The listing builds one solid part. Answer for the finished solid, in the listing's coordinates (mm). A direction names the side the tool comes from. Round coordinates to 2 decimals unless told otherwise and drop trailing zeros. Write each loop counter-clockwise with the first axis right and the second up, starting at its lowest first coordinate (ties: lowest second). Pieces come first, ordered by that corner, then holes. Notation, with made-up numbers: (-38, 76) - (1, 76) arc R24 ccw to (1, 90) - close; hole circle Ø11 at (80.25, 69.25). An arc over 180 degrees is marked (long way). Return JSON: item names as keys, results as strings. Group by question number.
(1) Determine the mould class of faces 1 (the cylindrical face through (54.46, 6.09, -1.48)), 2 (the flat face through (0, 0, -47)), 3 (the flat face through (59, 6, -3)) for opening direction Y: +Y half, -Y half, draft (parallel to the pull), parting line (faces both ways), or undercut.
(2) Section A-A, the plane y = 6 is taken. Write down the section's boundary in (x, z), then the cut area to 3 significant figures.
(3) Which of the six approach directions +Z, -Z, +X, -X, +Y, -Y give full straight-line access (tool end or side, diameter ignored) to faces 4 (the flat face through (-59, 6, -3)), 5 (the flat face through (-61.5, 6, -2))?
(4) Section C-C, the plane x = 0 is taken. Write down the section's boundary in (y, z), then the cut area to 3 significant figures.
(5) Find the intervals of material crossed by line 1 along Z through (x, y) = (57, 8); line 2 along X through (y, z) = (9, -1.5); line 3 along X through (y, z) = (6, -6), in increasing order. Write a range as [from, to].
(6) Section D-D, the plane x = 28 is taken. Write down the section's boundary in (y, z).
(7) Section B-B, the plane z = -24 is taken. Write down the section's boundary in (x, y).
(8) Each of these flat-tipped pins is pushed along its axis until it touches: pin 1 (3 mm diameter, centred on x = 22, y = 2.5, fed in from +Z); pin 2 (1.5 mm diameter, centred on x = 13, y = 8.5, fed in from -Z); pin 3 (2 mm diameter, centred on y = 8.5, z = -27, fed in from +X). Where does it stop, or does it pass through?
```python
from build123d import *

# Parameters (mm, degrees)
SKETCH1_R           = 46.5
BOSS_EXTRUDE1_DEPTH = 12
SKETCH2_R           = 2
CUT_EXTRUDE1_DEPTH  = 12
SKETCH3_W           = 95
SKETCH3_H           = 5
BOSS_EXTRUDE2_DEPTH = 12
MOVE_FACE1_BY       = 3
MOVE_FACE2_BY       = 3
MOVE_FACE2_2_BY     = 3
SKETCH4_R           = 2
CUT_EXTRUDE2_DEPTH  = 114.80355882
CUT_EXTRUDE3_DEPTH  = 2
FILLET1_R           = 1
FILLET2_R           = 1


with BuildPart() as part:
    # Sketch1 → Boss-Extrude1 (new body)
    with BuildSketch(Plane(origin=(0, 0, 0), x_dir=(1, 0, 0), z_dir=(0, 1, 0))):
        with BuildLine():
            Line((61.5, -3), (61.5, 3))
            Line((61.5, 3), (51.412547107, 3))
            ThreePointArc((51.412547107, 3), (0, 51.5), (-51.412547107, 3))
            Line((-51.412547107, 3), (-61.5, 3))
            Line((-61.5, 3), (-61.5, -3))
            Line((-61.5, -3), (-51.412547107, -3))
            ThreePointArc((-51.412547107, -3), (0, -51.5), (51.412547107, -3))
            Line((51.412547107, -3), (61.5, -3))
        make_face()
        with Locations(Location((0, 0, 0), (0, 0, 270))):
            Circle(SKETCH1_R, mode=Mode.SUBTRACT)
    extrude(amount=BOSS_EXTRUDE1_DEPTH)

    # Sketch2 → Cut-Extrude1 (cut)
    with BuildSketch(Plane.XY.offset(3)):
        with Locations((56.456273553, 6)):
            Circle(SKETCH2_R)
        with Locations((-56.456273553, 6)):
            Circle(SKETCH2_R)
    extrude(amount=-CUT_EXTRUDE1_DEPTH, mode=Mode.SUBTRACT)


with BuildPart() as body_2:
    # Split1: the piece on the far side of the plane
    add(part.part)
    split(bisect_by=Plane.XY, keep=Keep.BOTTOM)

    # Fillet2
    fillet2_edges = [body_2.edges().sort_by_distance(p)[0] for p in [
        (51.412547107, 6, -3),
        (-51.412547107, 6, -3),
    ]]
    fillet(fillet2_edges, radius=FILLET2_R)


with BuildPart() as part_1:
    add(part.part)

    # Split1
    split(bisect_by=Plane.XY, keep=Keep.TOP)

    # Sketch3 → Boss-Extrude2 (add)
    with BuildSketch(Plane(origin=(0, 12, 0), x_dir=(1, 0, 0), z_dir=(0, 1, 0))):
        with Locations((0, -49)):
            Rectangle(SKETCH3_W, SKETCH3_H)
    extrude(amount=-BOSS_EXTRUDE2_DEPTH)

    # Move Face1: a face moved inward by 3.0
    extrude(part_1.faces().sort_by_distance((0, 6, 51.5))[0], amount=MOVE_FACE1_BY, dir=(0, 0, -1), mode=Mode.SUBTRACT)

    # Move Face2: a face moved outward by 3.0
    extrude(part_1.faces().sort_by_distance((34.817971811, 6, 46.5))[0], amount=MOVE_FACE2_BY, dir=(0, 0, -1))

    # Move Face2 2: a face moved outward by 3.0
    extrude(part_1.faces().sort_by_distance((-34.817971811, 6, 46.5))[0], amount=MOVE_FACE2_2_BY, dir=(0, 0, -1))

    # Sketch4 → Cut-Extrude2 (cut, through all)
    with BuildSketch(Plane(origin=(0, 0, 43.5), x_dir=(-1, 0, 0), z_dir=(0, 0, -1))):
        with Locations((44.5, 6)):
            Circle(SKETCH4_R)
    cut_extrude2 = extrude(amount=-CUT_EXTRUDE2_DEPTH, mode=Mode.SUBTRACT)

    # Sketch5 → Cut-Extrude3 (cut)
    with BuildSketch(Plane(origin=(0, 0, 43.5), x_dir=(-1, 0, 0), z_dir=(0, 0, -1))):
        with BuildLine():
            Line((47.5, 12), (42.69457877, 9.569377282))
            ThreePointArc((42.69457877, 9.569377282), (40.5, 6), (42.69457877, 2.430622718))
            Line((42.69457877, 2.430622718), (47.5, 0))
            Line((47.5, 0), (47.5, 12))
        make_face()
    cut_extrude3 = extrude(amount=-CUT_EXTRUDE3_DEPTH, mode=Mode.SUBTRACT)

    # Mirror1: Cut-Extrude2, Cut-Extrude3 across plane
    add(cut_extrude2.mirror(Plane(origin=(0, 0, 0), x_dir=(0, 0, 1), z_dir=(1, 0, 0))), mode=Mode.SUBTRACT)
    add(cut_extrude3.mirror(Plane(origin=(0, 0, 0), x_dir=(0, 0, 1), z_dir=(1, 0, 0))), mode=Mode.SUBTRACT)

    # Fillet1
    fillet1_edges = [part_1.edges().sort_by_distance(p)[0] for p in [
        (47.5, 0, 44.5),
        (47.5, 12, 44.5),
        (51.412547107, 6, 3),
        (-51.412547107, 6, 3),
        (27.568097504, 6, 43.5),
        (-47.5, 0, 44.5),
        (-27.568097504, 6, 43.5),
        (-47.5, 12, 44.5),
    ]]
    fillet(fillet1_edges, radius=FILLET1_R)


solid = body_2.part
```
Working result:
{
 "1": {"face 1": "undercut", "face 2": "-Y half", "face 3": "draft"},
 "2": {"outline": "(-61.5, -3) - (-58.46, -3) - (-58.46, 0) - (-61.5, 0) - close; (-54.46, -3) - (-52.35, -3) arc R1 cw to (-51.35, -3.92) arc R51.5 ccw to (51.35, -3.92) arc R1 cw to (52.35, -3) - (54.46, -3) - (54.46, 0) - (46.5, 0) arc R46.5 cw to (-46.5, 0) - (-54.46, 0) - close; (58.46, -3) - (61.5, -3) - (61.5, 0) - (58.46, 0) - close", "area": "806 mm^2"},
 "3": {"face 4": "-Z, -X, +Y, -Y", "face 5": "+Z, -Z, -X, +Y, -Y"},
 "4": {"outline": "(0, -51.5) - (12, -51.5) - (12, -46.5) - (0, -46.5) - close", "area": "60.0 mm^2"},
 "5": {"line 1": "z = [-3, 0]", "line 2": "x = [-61.5, -46.48], [46.48, 61.5]", "line 3": "x = [-51.15, -46.11], [46.11, 51.15]"},
 "6": {"outline": "(0, -43.22) - (12, -43.22) - (12, -37.12) - (0, -37.12) - close"},
 "7": {"outline": "(-45.57, 0) - (-39.83, 0) - (-39.83, 12) - (-45.57, 12) - close; (39.83, 0) - (45.57, 0) - (45.57, 12) - (39.83, 12) - close"},
 "8": {"pin 1": "stops at z = -40.12", "pin 2": "stops at z = -50.02", "pin 3": "stops at x = 44.46"}
}
